Input: part model. Units: mm. Frame: model coordinates. Face numbers are marked on the shaded views. A direction names the side the tool comes from. Give positions to 0.01 mm unless a question says otherwise; leave off trailing zeros. Write each loop counter-clockwise with the first axis right and the second up, starting at its lowest first coordinate (ties: lowest second). Pieces come first, ordered by that corner, then holes. Notation, with made-up numbers: (-0.5, 74.25) -> (4.5, 74.25) arc R18 ccw to (4.5, 105.25) -> close; hole circle Ø11 at (54.5, -29.75). An arc over 180 degrees is marked (long way). Return JSON: item names as keys, results as strings. Group by question number.
Item 1: Section A-A, the plane y = 10. Return loops of the section in (x, z).
Item 2: Pin query (flat end, axial travel): P1, Ø2.5, axis at x = 0, z = 23, coming from the +Y side; P2, Ø4.5, axis at x = -13, y = -3.5, coming from the +Z side; P3, Ø8.5, axis at y = 6.5, z = 21, coming from the +X side; P4, Ø5, axis at y = 7, z = 28.5, coming from the -X side. Return the tip coordinate at first contact, or that it passes through.
Item 3: Section B-B, the plane y = 0. Return loops of the section in (x, z) (3 decimals), then the cut area to 3 significant figures.
Item 4: Line query: line 1 (Y direction, x = 16.5, z = 2.1); line 2 (X direction, y = -7.5, z = 4); line 3 (X direction, y = 0, z = 31). Output: solid intervals per line, ascending. Write a range as [from, to].
Item 5: Section D-D, the plane y = -6. Return loops of the section in (x, z).
Item 6: Set-up query: the marked faces 1, 2, 3 and 4. Return all of +Z, -Z, +X, -X, +Y, -Y with unobstructed straight access to the full face (end or side cutting, diameter ignored); none if empty.
Item 7: Section C-C, the plane x = 0. Return loops of the section in (y, z) (3 decimals), then the cut area to 3 significant figures.
Item 8: Mould query, pull axis Y, two halves, no side actions, for the marked faces 5, 6, 7 and 8. Classes: released by +Y, released by -Y, zero draft, split by the parting line, or undercut.
from build123d import *

# Parameters (mm, degrees)
SKETCH1_W                   = 45
SKETCH1_H                   = 30
BASE_DEPTH                  = 5
SKETCH2_W                   = 10
SKETCH2_H                   = 30
BOSS_EXTRUDE2_DEPTH         = 30
SKETCH3_R                   = 5
CUT_EXTRUDE3_DEPTH          = 10
SKETCH9_R                   = 3
SCREW_DEPTH                 = 5
SKETCH10_R                  = 3
TOP_HOLE_DEPTH              = 15
SKETCH11_R                  = 1.5
BOTTOM_HOLE_DEPTH           = 15
FILLET1_R                   = 2
FILLET2_R                   = 2
M4_TAPPED_HOLE3_D           = 3.3
M4_TAPPED_HOLE3_DEPTH       = 10.1
M4_TAPPED_HOLE3_CSINK_D     = 4.05
M4_TAPPED_HOLE3_CSINK_ANGLE = 90
M4_TAPPED_HOLE3_TIP         = 0.991420021


with BuildPart() as part:
    # Sketch1 → Base (new body)
    with BuildSketch(Plane.XY):
        Rectangle(SKETCH1_W, SKETCH1_H)
    extrude(amount=BASE_DEPTH)

    # Sketch2 → Boss-Extrude2 (add)
    with BuildSketch(Plane.XY.offset(5)):
        Rectangle(SKETCH2_W, SKETCH2_H)
    extrude(amount=BOSS_EXTRUDE2_DEPTH)

    # Sketch3 → Cut-Extrude3 (cut)
    with BuildSketch(Plane.ZY.offset(5)):
        with Locations((23, 0)):
            Circle(SKETCH3_R)
    extrude(amount=-CUT_EXTRUDE3_DEPTH, mode=Mode.SUBTRACT)

    # Sketch9 → Screw (cut)
    with BuildSketch(Plane.XY.offset(5)):
        with Locations((-16.5, 10)):
            Circle(SKETCH9_R)
        with Locations((-16.5, 0)):
            Circle(SKETCH9_R)
        with Locations((-16.5, -10)):
            Circle(SKETCH9_R)
        with Locations((16.5, -10)):
            Circle(SKETCH9_R)
        with Locations((16.5, 0)):
            Circle(SKETCH9_R)
        with Locations((16.5, 10)):
            Circle(SKETCH9_R)
    extrude(amount=-SCREW_DEPTH, mode=Mode.SUBTRACT)

    # Sketch10 → Top hole (cut)
    with BuildSketch(Plane(origin=(0, 15, 0), x_dir=(1, 0, 0), z_dir=(0, 1, 0))):
        with Locations((0, -23)):
            Circle(SKETCH10_R)
    extrude(amount=-TOP_HOLE_DEPTH, mode=Mode.SUBTRACT)

    # Sketch11 → Bottom hole (cut)
    with BuildSketch(Plane.XZ.offset(15)):
        with Locations((0, 23)):
            Circle(SKETCH11_R)
    extrude(amount=-BOTTOM_HOLE_DEPTH, mode=Mode.SUBTRACT)

    # Fillet1
    fillet1_edges = [part.edges().sort_by_distance(p)[0] for p in [
        (-5, 0, 5),
    ]]
    fillet(fillet1_edges, radius=FILLET1_R)

    # Fillet2
    fillet2_edges = [part.edges().sort_by_distance(p)[0] for p in [
        (5, 0, 5),
    ]]
    fillet(fillet2_edges, radius=FILLET2_R)

    # M4 Tapped Hole3
    with Locations(Plane.XY.offset(35)):
        with Locations((0, 0)):
            CounterSinkHole(M4_TAPPED_HOLE3_D / 2, M4_TAPPED_HOLE3_CSINK_D / 2, depth=M4_TAPPED_HOLE3_DEPTH, counter_sink_angle=M4_TAPPED_HOLE3_CSINK_ANGLE)
            with Locations((0, 0, -(M4_TAPPED_HOLE3_DEPTH + M4_TAPPED_HOLE3_TIP / 2))):  # 118° drill point
                Cone(0, M4_TAPPED_HOLE3_D / 2, M4_TAPPED_HOLE3_TIP, mode=Mode.SUBTRACT)


solid = part.part
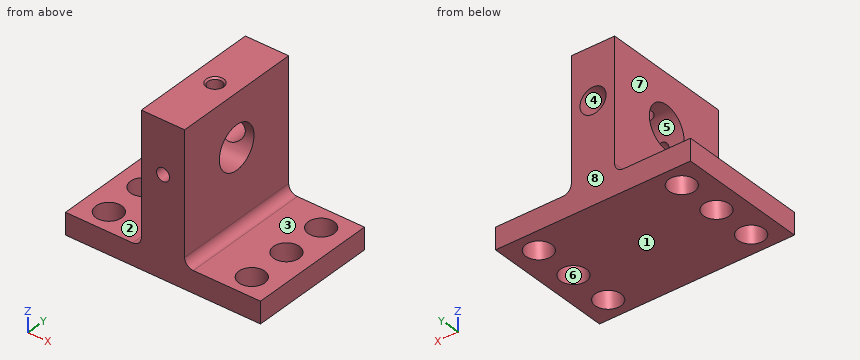
Answer below:
{
 "1": {"outline": "(-22.5, 0) -> (-19.5, 0) -> (-19.5, 5) -> (-22.5, 5) -> close; (-13.5, 0) -> (13.5, 0) -> (13.5, 5) -> (7, 5) arc R2 cw to (5, 7) -> (5, 35) -> (-5, 35) -> (-5, 7) arc R2 cw to (-7, 5) -> (-13.5, 5) -> close; (19.5, 0) -> (22.5, 0) -> (22.5, 5) -> (19.5, 5) -> close; hole circle Ø6 at (0, 23)"},
 "2": {"P1": "passes through", "P2": "stops at z = 5", "P3": "stops at x = 5", "P4": "stops at x = -5"},
 "3": {"outline": "(-22.5, 0) -> (-19.5, 0) -> (-19.5, 5) -> (-22.5, 5) -> close; (-13.5, 0) -> (13.5, 0) -> (13.5, 5) -> (7, 5) arc R2 cw to (5, 7) -> (5, 18) -> (-5, 18) -> (-5, 7) arc R2 cw to (-7, 5) -> (-13.5, 5) -> close; (-5, 28) -> (-1.65, 28) -> (-1.65, 34.625) -> (-2.025, 35) -> (-5, 35) -> close; (1.65, 28) -> (5, 28) -> (5, 35) -> (2.025, 35) -> (1.65, 34.625) -> close; (19.5, 0) -> (22.5, 0) -> (22.5, 5) -> (19.5, 5) -> close", "area": "343 mm2"},
 "4": {"line 1": "y = [-15, -13], [-7, -3], [3, 7], [13, 15]", "line 2": "x = [-22.5, -18.16], [-14.84, 14.84], [18.16, 22.5]", "line 3": "x = [-5, -1.65], [1.65, 5]"},
 "5": {"outline": "(-22.5, 0) -> (22.5, 0) -> (22.5, 5) -> (7, 5) arc R2 cw to (5, 7) -> (5, 35) -> (-5, 35) -> (-5, 7) arc R2 cw to (-7, 5) -> (-22.5, 5) -> close; hole circle Ø3 at (0, 23)"},
 "6": {"face 1": "-Z, +X, -X, +Y, -Y", "face 2": "+Z, -X, +Y, -Y", "face 3": "+Z, +X, +Y, -Y", "face 4": "+Y"},
 "7": {"outline": "(-15, 0) -> (15, 0) -> (15, 20) -> (4, 20) arc R5 cw to (-4.77, 21.5) -> (-15, 21.5) -> close; (-15, 24.5) -> (-4.77, 24.5) arc R5 cw to (-1.65, 27.72) -> (-1.65, 34.625) -> (-2.025, 35) -> (-15, 35) -> close; (1.65, 27.72) arc R5 cw to (4, 26) -> (15, 26) -> (15, 35) -> (2.025, 35) -> (1.65, 34.625) -> close", "area": "856 mm2"},
 "8": {"face 5": "undercut", "face 6": "undercut", "face 7": "zero draft", "face 8": "released by +Y"}
}
